```python
from build123d import *
from build123d.topology import SkipClean

# Parameters (mm, degrees)
BOSS_EXTRU_3_DEPTH           = 3
ENL_V_MAT_EXTRU_1_DEPTH      = 63.157059132
ENL_V_MAT_EXTRU_1_DEPTH_BACK = 3
ENL_V_MAT_EXTRU_2_DEPTH      = 3
ESQUISSE5_W                  = 6
ESQUISSE5_H                  = 0.5
ENL_V_MAT_EXTRU_4_DEPTH      = 63.227405538


with BuildPart() as part:
    # Esquisse1 → Boss.-Extru.3 (new body)
    with BuildSketch(Plane.XY):
        with BuildLine():
            Line((43.5, 0), (0, 0))
            Line((0, 0), (0, -2.5))
            Line((0, -2.5), (-10, -2.5))
            Line((-10, -2.5), (-10, -4))
            Line((-10, -4), (2, -4))
            Line((2, -4), (2, -3.5))
            ThreePointArc((2, -3.5), (2.292893219, -2.792893219), (3, -2.5))
            Line((3, -2.5), (41, -2.5))
            ThreePointArc((41, -2.5), (41.707106781, -2.792893219), (42, -3.5))
            Line((42, -3.5), (42, -4.5))
            Line((42, -4.5), (54, -4.5))
            Line((54, -4.5), (54, -4.330127019))
            ThreePointArc((54, -4.330127019), (54.5, -3.464101615), (55.5, -3.464101615))
            ThreePointArc((55.5, -3.464101615), (59.5, -3.464101615), (61.5, 0))
            Line((61.5, 0), (59, 0))
            ThreePointArc((59, 0), (57.5, -1.5), (56, 0))
            Line((56, 0), (53, 0))
            Line((53, 0), (53, -2.5))
            Line((53, -2.5), (49.5, -2.5))
            Line((49.5, -2.5), (49.5, -3))
            Line((49.5, -3), (43.5, -3))
            Line((43.5, -3), (43.5, 0))
        make_face()
    boss_extru_3 = extrude(amount=BOSS_EXTRU_3_DEPTH)

    # Symétrie2: Boss.-Extru.3 across plane
    with SkipClean():  # the faces are left unmerged after this step: merging them gives an invalid solid
        add(boss_extru_3.mirror(Plane(origin=(0, 0, 3), x_dir=(0, 0, 1), z_dir=(0, 1, 0))))

    # Esquisse2 → Enlèv. mat.-Extru.1 (cut, two sides: drawn at the far end of the back side and taken through both)
    with SkipClean():  # the faces are left unmerged after this step: merging them gives an invalid solid
        with BuildSketch(Plane(origin=(0, 4, 0), x_dir=(1, 0, 0), z_dir=(0, 1, 0)).offset(-ENL_V_MAT_EXTRU_1_DEPTH_BACK)):
            with BuildLine():
                Line((-9.2, -0.95), (-8.3, -0.95))
                ThreePointArc((-8.3, -0.95), (-7.75, -1.5), (-8.3, -2.05))
                Line((-8.3, -2.05), (-9.2, -2.05))
                ThreePointArc((-9.2, -2.05), (-9.75, -1.5), (-9.2, -0.95))
            make_face()
        extrude(amount=ENL_V_MAT_EXTRU_1_DEPTH + ENL_V_MAT_EXTRU_1_DEPTH_BACK, mode=Mode.SUBTRACT)

    # Esquisse3 → Enlèv. mat.-Extru.2 (cut)
    with SkipClean():  # the faces are left unmerged after this step: merging them gives an invalid solid
        with BuildSketch(Plane.XZ.offset(4)):
            with BuildLine():
                Line((-9.4, 2.05), (-8.3, 2.05))
                ThreePointArc((-8.3, 2.05), (-7.75, 1.5), (-8.3, 0.95))
                Line((-8.3, 0.95), (-9.4, 0.95))
                ThreePointArc((-9.4, 0.95), (-9.95, 1.5), (-9.4, 2.05))
            make_face()
        extrude(amount=-ENL_V_MAT_EXTRU_2_DEPTH, mode=Mode.SUBTRACT)

    # Esquisse5 → Enlèv. mat.-Extru.4 (cut, through all)
    with SkipClean():  # the faces are left unmerged after this step: merging them gives an invalid solid
        with BuildSketch(Plane.XZ.offset(4.5)):
            Polygon((42, 2.5), (42, 3), (3, 3), (3, 2.5), (41, 2.5), align=None)
            Polygon((3, 0), (42, 0), (42, 0.5), (41, 0.5), (3, 0.5), align=None)
            with Locations((58.5, 2.75)):
                Rectangle(ESQUISSE5_W, ESQUISSE5_H)
            with Locations((58.5, 0.25)):
                Rectangle(ESQUISSE5_W, ESQUISSE5_H)
        extrude(amount=-ENL_V_MAT_EXTRU_4_DEPTH, mode=Mode.SUBTRACT)


solid = part.part
```
CAD build for the part. Positions are in the model's coordinates, mm. A direction names the side the tool comes from. Coordinates: 2 decimals unless noted, no trailing zeros. Order: outer loops, then holes, each group sorted by start corner. A loop starts at its lowest first (then second) coordinate and runs counter-clockwise, first axis right, second up. Notation, with made-up numbers: (1.25, 32.5) -> (27.25, 32.5) arc R32 ccw to (27.25, 60.5) -> close; hole circle Ø5 at (66.5, 46.5). An arc over 180 degrees is marked (long way). Use one line per item in the form item = value. Start each with the question number.
1) Pull direction Y, two halves, no side cores. Call faces 4 (the flat face through (-4, 4, 1)), 5 (the flat face through (-9, -3, 2.05)), 6 (the flat face through (0, 0, 1)): +Y half, -Y half, draft (parallel to the pull), parting line (faces both ways), or undercut.
2) Band-saw the part on A-A on x = 57.5. Give the cut face in (y, z).
3) Drop flat-ended pins along their axis: pin 1 (1.5 mm diameter, centred on x = -6.5, z = 1, fed in from +Y); pin 2 (4 mm diameter, centred on x = 12.5, y = -0.5, fed in from -Z); pin 3 (1 mm diameter, centred on x = 34.5, z = 2, fed in from -Y). Give the stop position or say it passes through.
4) Band-saw the part on B-B on y = 0.75. Give the cut face in (x, z), then the cut area to 3 significant figures.
5) Drill centre lines: L1, parallel to X at y = 1, z = 2.6; L2, parallel to Y at x = 57.5, z = 1.7; L3, parallel to X at y = 0.25, z = 1.8. Where is each one in solid material? Low to high. Write a range as [from, to].
6) Tool access for faces 1 (the flat face through (23, 0, 0.5)), 2 (the flat face through (22, 0, 2.5)), 3 (the flat face through (53, 0, 1)): list every direction of +Z, -Z, +X, -X, +Y, -Y with a clear straight run to the whole face (end or side of a thin tool).
7) Band-saw the part on C-C on x = 33. Give the cut face in (y, z).
Entries:
q1.face_4 = +Y half
q1.face_5 = draft
q1.face_6 = undercut
q2.outline = (-4, 0.5) -> (-1.5, 0.5) -> (-1.5, 2.5) -> (-4, 2.5) -> close; (1.5, 0.5) -> (4, 0.5) -> (4, 2.5) -> (1.5, 2.5) -> close
q3.pin_1 = 4
q3.pin_2 = 0.5
q3.pin_3 = -2.5
q4.outline = (0, 0) -> (3, 0) -> (3, 0.5) -> (42, 0.5) -> (42, 0) -> (43.5, 0) -> (43.5, 3) -> (42, 3) -> (42, 2.5) -> (3, 2.5) -> (3, 3) -> (0, 3) -> close; (53, 0) -> (55.5, 0) -> (55.5, 0.5) -> (56.2, 0.5) -> (56.2, 2.5) -> (55.5, 2.5) -> (55.5, 3) -> (53, 3) -> close; (58.8, 0.5) -> (61.43, 0.5) -> (61.43, 2.5) -> (58.8, 2.5) -> close
q4.area = 106 mm2
q5.L1 = [0, 3], [42, 43.5], [53, 55.5]
q5.L2 = [-4, -1.5], [1.5, 4]
q5.L3 = [0, 43.5], [53, 56.02], [58.98, 61.49]
q6.face_1 = -Z, +Y, -Y
q6.face_2 = +Z, +Y, -Y
q6.face_3 = +Z, -Z
q7.outline = (-2.5, 0.5) -> (2.5, 0.5) -> (2.5, 2.5) -> (-2.5, 2.5) -> close
